For this review, take the finished solid that the model builds, in its own axes (mm). Face numbers are marked on the shaded views. A direction names the side the tool comes from. Give positions to 0.01 mm unless a question says otherwise; leave off trailing zeros. Order: outer loops, then holes, each group sorted by start corner. A loop starts at its lowest first (then second) coordinate and runs counter-clockwise, first axis right, second up. Notation, with made-up numbers: (46, 74) -> (88, 74) arc R22 ccw to (88, 80) -> close; hole circle Ø2 at (2, 12). An arc over 180 degrees is marked (long way). Return JSON: item names as keys, results as strings. Group by question number.
1) Add section D-D (z = 2.75). Give the boundary of the cut face in (x, y), then the cut area to 3 significant figures.
2) The part is to be moulded in two halves that separate along X. For the marked faces 1, 2, 3 and 4, say which applies: released by +X, released by -X, zero draft, split by the parting line, or undercut.
3) Insertion check: P1, Ø3.5, axis at x = -13.66, y = -16.49, coming from the -Z side; P2, Ø8, axis at x = 22.5, y = 5, coming from the +Z side; P3, Ø2, axis at y = -5.5, z = 2, coming from the -X side; P4, Ø1.5, axis at y = -19, z = -1, coming from the -X side. Each pin has a flat end and moves straight along its axis. Give the tip position at first contact, or say it passes through.
4) To check wall thickness, follow line 1 along X through (y, z) = (11, 13.25); line 2 along X through (y, z) = (11, -0.5); line 3 along Z through (x, y) = (0, 4). State the ranges of each line that lie inside material, in increasing order.
5) Add section B-B (x = -14.5). Give the boundary of the cut face in (y, z), then the cut area to 3 significant figures.
6) Add section A-A (z = 13.5). Give the boundary of the cut face in (x, y), then the cut area to 3 significant figures.
7) Add section C-C (y = 11). State how many separate pieces and enclosed holes the cut face has, then the cut area to 3 significant figures.
8) For the marked faces 5 and 6, list the 3-axis set-ups (+Z, -Z, +X, -X, +Y, -Y) from which the entire face can be reached by the end or side of a thin tool; tool diameter is ignored.
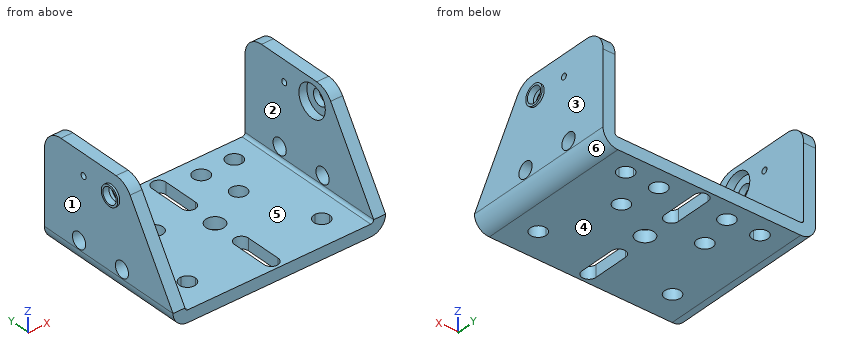
from build123d import *

# Parameters (mm, degrees)
ESBO_O1_W                        = 47.5
ESBO_O1_H                        = 39
FLANGE_BASE1_DEPTH               = 3
ESBO_O6_R                        = 2.3
CORTE_EXTRUS_O1_DEPTH            = 10
ARESTA_FLANGE1_STRIP_W           = 13.4732
ARESTA_FLANGE1_STRIP_H           = 3
ARESTA_FLANGE1_STRIP_CUT_DEPTH   = 39
ARESTA_FLANGE1_STRIP_2_W         = 13.4732
ARESTA_FLANGE1_STRIP_2_H         = 3
ARESTA_FLANGE1_STRIP_CUT_2_DEPTH = 39
ARESTA_FLANGE1_DEPTH             = 39
ARESTA_FLANGE1_BEND_DEPTH        = 39
ESBO_O13_R                       = 2
ESBO_O13_R_2                     = 0.75
CORTE_EXTRUS_O2_DEPTH            = 70
FILETE1_R                        = 5
ESBO_O14_R                       = 1.997873176
ESBO_O14_R_2                     = 2.026064888
ESBO_O14_R_3                     = 2
CORTE_EXTRUS_O4_DEPTH            = 15.5
BOSS_EXTRUDE1_START              = 0.5
SKETCH1_R                        = 2.5
SKETCH1_R_2                      = 2
BOSS_EXTRUDE1_DEPTH              = 0.5
SKETCH2_R                        = 4
CUT_EXTRUDE8_DEPTH               = 2
ESBO_O15_R                       = 2
CORTE_EXTRUS_O5_DEPTH            = 64.777464961


# Sheet-metal steps are written as plain solids
with BuildPart() as part:
    # Esboço1 → Flange-base1 (new body)
    with BuildSketch(Plane.XY):
        with Locations((3.243735783, -4.490936556)):
            Rectangle(ESBO_O1_W, ESBO_O1_H)
    extrude(amount=-FLANGE_BASE1_DEPTH)

    # Esboço6 → Corte-extrusão1 (cut)
    with BuildSketch(Plane.XY):
        with BuildLine():
            Line((-13.656264217, 8.009063444), (-13.656264217, 10.009063444))
            Line((-13.656264217, 10.009063444), (-11.656264217, 10.009063444))
            ThreePointArc((-11.656264217, 10.009063444), (-15.070477779, 11.423277006), (-13.656264217, 8.009063444))
        make_face()
        with BuildLine():
            Line((-11.656264217, 10.009063444), (-13.656264217, 10.009063444))
            Line((-13.656264217, 10.009063444), (-13.656264217, 8.009063444))
            ThreePointArc((-13.656264217, 8.009063444), (-12.242050654, 8.594849882), (-11.656264217, 10.009063444))
        make_face()
        with BuildLine():
            ThreePointArc((-11.656264217, -16.490936556), (-12.242050654, -15.076722994), (-13.656264217, -14.490936556))
            Line((-13.656264217, -14.490936556), (-13.656264217, -16.490936556))
            Line((-13.656264217, -16.490936556), (-11.656264217, -16.490936556))
        make_face()
        with BuildLine():
            Line((-13.656264217, -16.490936556), (-13.656264217, -14.490936556))
            ThreePointArc((-13.656264217, -14.490936556), (-15.070477779, -17.905150118), (-11.656264217, -16.490936556))
            Line((-11.656264217, -16.490936556), (-13.656264217, -16.490936556))
        make_face()
        with Locations((3.243735783, -4.490936556)):
            Circle(ESBO_O6_R)
        with BuildLine():
            Line((4.993735783, 10.009063444), (1.493735783, 10.009063444))
            Line((1.493735783, 10.009063444), (1.493735783, 3.523823043))
            ThreePointArc((1.493735783, 3.523823043), (3.243735783, 1.773823043), (4.993735783, 3.523823043))
            Line((4.993735783, 3.523823043), (4.993735783, 10.009063444))
        make_face()
        with BuildLine():
            Line((1.493735783, 12.523823043), (1.493735783, 10.009063444))
            Line((1.493735783, 10.009063444), (4.993735783, 10.009063444))
            Line((4.993735783, 10.009063444), (4.993735783, 12.523823043))
            ThreePointArc((4.993735783, 12.523823043), (3.243735783, 14.273823043), (1.493735783, 12.523823043))
        make_face()
        with BuildLine():
            Line((1.493735783, -12.505696155), (1.493735783, -16.490936556))
            Line((1.493735783, -16.490936556), (4.993735783, -16.490936556))
            Line((4.993735783, -16.490936556), (4.993735783, -12.505696155))
            ThreePointArc((4.993735783, -12.505696155), (3.243735783, -10.755696155), (1.493735783, -12.505696155))
        make_face()
        with BuildLine():
            Line((4.993735783, -16.490936556), (1.493735783, -16.490936556))
            Line((1.493735783, -16.490936556), (1.493735783, -21.505696155))
            ThreePointArc((1.493735783, -21.505696155), (3.243735783, -23.255696155), (4.993735783, -21.505696155))
            Line((4.993735783, -21.505696155), (4.993735783, -16.490936556))
        make_face()
        with BuildLine():
            ThreePointArc((22.143735783, -16.490936556), (21.557949346, -15.076722994), (20.143735783, -14.490936556))
            Line((20.143735783, -14.490936556), (20.143735783, -16.490936556))
            Line((20.143735783, -16.490936556), (18.143735783, -16.490936556))
            ThreePointArc((18.143735783, -16.490936556), (20.143735783, -18.490936556), (22.143735783, -16.490936556))
        make_face()
        with BuildLine():
            Line((20.143735783, -16.490936556), (20.143735783, -14.490936556))
            ThreePointArc((20.143735783, -14.490936556), (18.729522221, -15.076722994), (18.143735783, -16.490936556))
            Line((18.143735783, -16.490936556), (20.143735783, -16.490936556))
        make_face()
        with BuildLine():
            ThreePointArc((22.143735783, 10.009063444), (20.143735783, 12.009063444), (18.143735783, 10.009063444))
            Line((18.143735783, 10.009063444), (20.143735783, 10.009063444))
            Line((20.143735783, 10.009063444), (20.143735783, 8.009063444))
            ThreePointArc((20.143735783, 8.009063444), (21.557949346, 8.594849882), (22.143735783, 10.009063444))
        make_face()
        with BuildLine():
            Line((20.143735783, 10.009063444), (18.143735783, 10.009063444))
            ThreePointArc((18.143735783, 10.009063444), (18.729522221, 8.594849882), (20.143735783, 8.009063444))
            Line((20.143735783, 8.009063444), (20.143735783, 10.009063444))
        make_face()
    extrude(amount=-CORTE_EXTRUS_O1_DEPTH, mode=Mode.SUBTRACT)

    # Aresta-Flange1 strip (across the edge) → Aresta-Flange1 strip cut (cut)
    with BuildSketch(Plane(origin=(26.993735783, -23.990936556, 0), x_dir=(-1, 0, 0), z_dir=(0, 1, 0))):
        with Locations((-6, -1.5)):
            Rectangle(ARESTA_FLANGE1_STRIP_W, ARESTA_FLANGE1_STRIP_H)
    extrude(amount=ARESTA_FLANGE1_STRIP_CUT_DEPTH, mode=Mode.SUBTRACT)

    # Aresta-Flange1 strip 2 (across the edge) → Aresta-Flange1 strip cut 2 (cut)
    with BuildSketch(Plane(origin=(-20.506264217, 15.009063444, 0), x_dir=(1, 0, 0), z_dir=(0, -1, 0))):
        with Locations((-6, -1.5)):
            Rectangle(ARESTA_FLANGE1_STRIP_2_W, ARESTA_FLANGE1_STRIP_2_H)
    extrude(amount=ARESTA_FLANGE1_STRIP_CUT_2_DEPTH, mode=Mode.SUBTRACT)

    # Aresta-Flange1 section (across the edge) → Aresta-Flange1 (add)
    with BuildSketch(Plane(origin=(26.993735783, -23.990936556, 0), x_dir=(-1, 0, 0), z_dir=(0, 1, 0))):
        with BuildLine():
            Line((-3, 0.7366), (-3, 24))
            Line((-3, 24), (0, 24))
            Line((0, 24), (0, 0.7366))
            ThreePointArc((0, 0.7366), (0.215745145, 0.215745145), (0.7366, 0))
            Line((0.7366, 0), (0.7366, -3))
            ThreePointArc((0.7366, -3), (-1.905575199, -1.905575199), (-3, 0.7366))
        make_face()
    extrude(amount=ARESTA_FLANGE1_DEPTH)

    # Aresta-Flange1 section 2 (across the edge) → Aresta-Flange1 bend (add)
    with BuildSketch(Plane(origin=(-20.506264217, 15.009063444, 0), x_dir=(1, 0, 0), z_dir=(0, -1, 0))):
        with BuildLine():
            Line((-3, 0.7366), (-3, 24))
            Line((-3, 24), (0, 24))
            Line((0, 24), (0, 0.7366))
            ThreePointArc((0, 0.7366), (0.215745145, 0.215745145), (0.7366, 0))
            Line((0.7366, 0), (0.7366, -3))
            ThreePointArc((0.7366, -3), (-1.905575199, -1.905575199), (-3, 0.7366))
        make_face()
    extrude(amount=ARESTA_FLANGE1_BEND_DEPTH)

    # Esboço13 → Corte-extrusão2 (cut)
    with BuildSketch(Plane.ZY.offset(23.506264217)):
        with Locations((18.734737, -5.325205188)):
            Circle(ESBO_O13_R)
        with Locations((18.734737, 3.124794812)):
            Circle(ESBO_O13_R_2)
        Polygon((0.7366, -23.990936556), (24, -23.990936556), (24, -9.490936556), align=None)
    extrude(amount=-CORTE_EXTRUS_O2_DEPTH, mode=Mode.SUBTRACT)

    # Filete1
    filete1_edges = [part.edges().sort_by_distance(p)[0] for p in [
        (28.493735783, 15.009063444, 24),
        (-22.006264217, 15.009063444, 24),
        (-22.006264217, -9.490936556, 24),
        (28.493735783, -9.490936556, 24),
    ]]
    fillet(filete1_edges, radius=FILETE1_R)

    # Esboço14 → Corte-extrusão4 (cut)
    with BuildSketch(Plane.XY):
        with Locations((-5.331264217, 10.009063444)):
            Circle(ESBO_O14_R)
        with Locations((11.818735783, 10.009063444)):
            Circle(ESBO_O14_R_2)
        with Locations((13.743735783, 1.009063444)):
            Circle(ESBO_O14_R_3)
        with Locations((-7.256264217, 1.009063444)):
            Circle(ESBO_O14_R_3)
    extrude(amount=-CORTE_EXTRUS_O4_DEPTH, mode=Mode.SUBTRACT)

    # Sketch1 → Boss-Extrude1 (add)
    with BuildSketch(Plane.ZY.offset(23.506264217).offset(BOSS_EXTRUDE1_START)):
        with Locations(Location((18.734737, -5.325205188, 0), (0, 0, 180))):
            Circle(SKETCH1_R)
        with Locations((18.734737, -5.325205188)):
            Circle(SKETCH1_R_2, mode=Mode.SUBTRACT)
    boss_extrude1 = extrude(amount=-BOSS_EXTRUDE1_DEPTH)

    # Sketch2 → Cut-Extrude8 (cut)
    with BuildSketch(Plane(origin=(-20.506264217, 0, 0), x_dir=(0, 0, -1), z_dir=(1, 0, 0))):
        with Locations((-18.734737, -5.325205188)):
            Circle(SKETCH2_R)
    cut_extrude8 = extrude(amount=-CUT_EXTRUDE8_DEPTH, mode=Mode.SUBTRACT)

    # Mirror1: Boss-Extrude1, Cut-Extrude8 across plane
    add(boss_extrude1.mirror(Plane.ZY.offset(-3.243735783)))
    add(cut_extrude8.mirror(Plane.ZY.offset(-3.243735783)), mode=Mode.SUBTRACT)

    # Esboço15 → Corte-extrusão5 (cut, through all)
    with BuildSketch(Plane.ZY.offset(23.506264217)):
        with Locations((2.9366, 4.509063444)):
            Circle(ESBO_O15_R)
        with Locations((2.9366, -8.490936556)):
            Circle(ESBO_O15_R)
    extrude(amount=-CORTE_EXTRUS_O5_DEPTH, mode=Mode.SUBTRACT)


solid = part.part
Evaluation:
{
 "1": {"outline": "(-23.51, -22.74) -> (-20.51, -22.74) -> (-20.51, -10.48) -> (-23.51, -10.48) -> close; (-23.51, -6.5) -> (-20.51, -6.5) -> (-20.51, 2.52) -> (-23.51, 2.52) -> close; (-23.51, 6.5) -> (-20.51, 6.5) -> (-20.51, 15.01) -> (-23.51, 15.01) -> close; (26.99, -22.74) -> (29.99, -22.74) -> (29.99, -10.48) -> (26.99, -10.48) -> close; (26.99, -6.5) -> (29.99, -6.5) -> (29.99, 2.52) -> (26.99, 2.52) -> close; (26.99, 6.5) -> (29.99, 6.5) -> (29.99, 15.01) -> (26.99, 15.01) -> close", "area": "179 mm^2"},
 "2": {"face 1": "released by -X", "face 2": "undercut", "face 3": "released by +X", "face 4": "zero draft"},
 "3": {"P1": "through", "P2": "z = 0.04", "P3": "x = -23.51", "P4": "x = -23.37"},
 "4": {"line 1": "-23.51 to -20.51, 26.99 to 29.99", "line 2": "-23.3 to -15.39, -11.92 to -7.07, -3.6 to 1.49, 4.99 to 10.05, 13.59 to 18.41, 21.88 to 29.78", "line 3": "-3 to 0"},
 "5": {"outline": "(-23.99, -3) -> (-18.3, -3) -> (-18.3, 0) -> (-23.99, 0) -> close; (-14.68, -3) -> (8.2, -3) -> (8.2, 0) -> (-14.68, 0) -> close; (11.82, -3) -> (15.01, -3) -> (15.01, 0) -> (11.82, 0) -> close", "area": "95.2 mm^2"},
 "6": {"outline": "(-23.51, -16.04) -> (-20.51, -16.04) -> (-20.51, 15.01) -> (-23.51, 15.01) -> close; (26.99, -16.04) -> (29.99, -16.04) -> (29.99, 15.01) -> (26.99, 15.01) -> close", "area": "186 mm^2"},
 "7": {"separate pieces": "6", "enclosed holes": "0", "area": "246 mm^2"},
 "8": {"face 5": "+Z, +Y, -Y", "face 6": "-Z, +X, +Y, -Y"}
}
